The figure shows three views and two pictorial views of one solid part (mm, origin at its lowest corner). Answer the questions. A direction names the side the tool comes from. Round coordinates to 2 decimals unless told otherwise and drop trailing zeros. Write each loop counter-clockwise with the first axis right and the second up, starting at its lowest first coordinate (ties: lowest second). Pieces come first, ordered by that corner, then holes.
Item 1: Find section C-C on y = 20.25. Give the vertices of the cut face in (x, z) (1 decimal).
Item 2: For a pull along Y with two mould halves and no side action, classify the marked faces 1, 2, 3 and 4 as +Y half, -Y half, draft (parallel to the pull), parting line (faces both ways), or undercut.
Item 3: Find the intervals of material crossed by probe 1 along Y at (x, z) = (3.81, 1.25); probe 2 along X at (y, z) = (9.75, 10) (1 decimal); probe 3 along X at (y, z) = (10.5, 3.75) (1 decimal), in increasing order.
Item 4: Each of these flat-tipped pins is pushed along its axis until it touches: pin 1 (2.5 mm diameter, centred on x = 3.81, y = 5.4, fed in from -Z); pin 2 (1.5 mm diameter, centred on x = 31, y = 10, fed in from +Z); pin 3 (4 mm diameter, centred on y = 11.5, z = 13.5, fed in from -X). Where does it stop, or does it pass through?
Item 5: Find section B-B on x = 3.81. Give the vertices of the cut face in (y, z).
Item 6: Find section A-A on z = 8.25. Give the vertices of the cut face in (x, y) (1 decimal), then the cut area to 3 significant figures.
Item 7: Find section D-D on x = 30.5. Give the vertices of the cut face in (y, z), then the cut area to 3 significant figures.
Item 8: A tool of negligible diameter and unlimited length cuts with its end or side. For the marked faces 5, 6 and 7, from which of +Z, -Z, +X, -X, +Y, -Y can it reach the whole face along a straight path? Write none if from no direction.
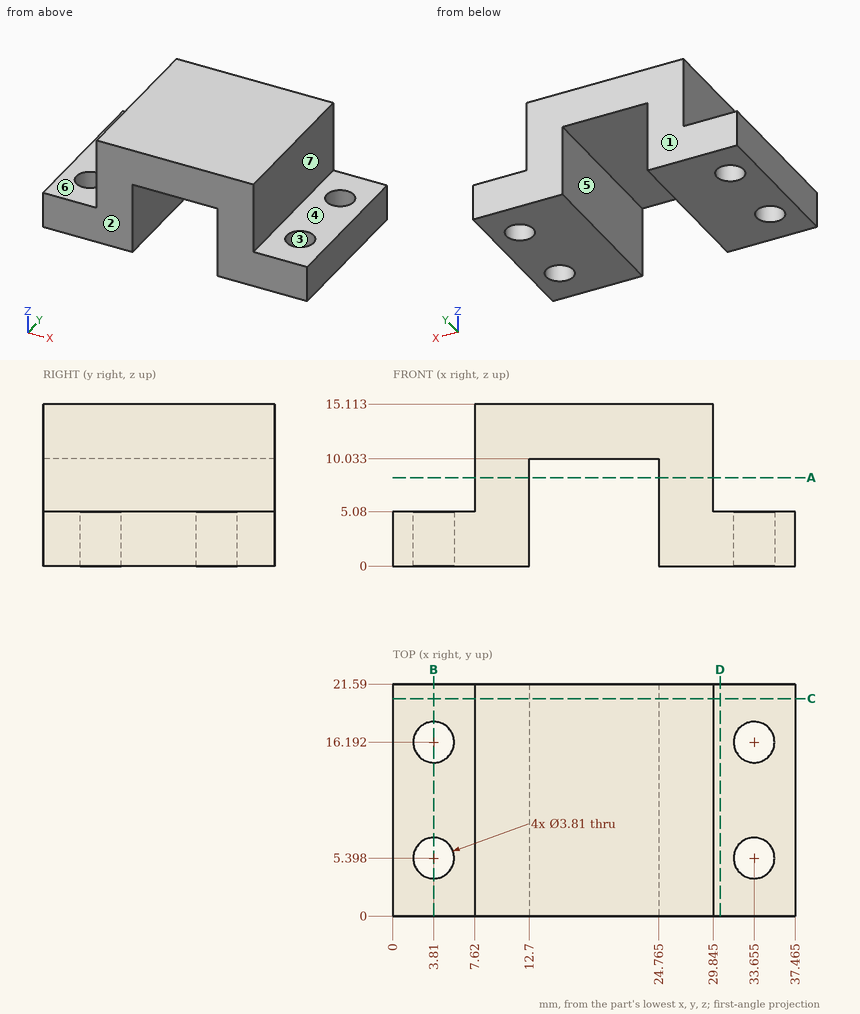
Check values:
1. outline: (0, 0) - (12.7, 0) - (12.7, 10) - (24.8, 10) - (24.8, 0) - (37.5, 0) - (37.5, 5.1) - (29.8, 5.1) - (29.8, 15.1) - (7.6, 15.1) - (7.6, 5.1) - (0, 5.1) - close
2. face 1: +Y half
2. face 2: -Y half
2. face 3: undercut
2. face 4: draft
3. probe 1: y = 0 to 3.49, 7.3 to 14.29, 18.1 to 21.59
3. probe 2: x = 7.6 to 12.7, 24.8 to 29.8
3. probe 3: x = 0 to 12.7, 24.8 to 37.5
4. pin 1: passes through
4. pin 2: stops at z = 5.08
4. pin 3: stops at x = 7.62
5. outline: (0, 0) - (3.49, 0) - (3.49, 5.08) - (0, 5.08) - close; (7.3, 0) - (14.29, 0) - (14.29, 5.08) - (7.3, 5.08) - close; (18.1, 0) - (21.59, 0) - (21.59, 5.08) - (18.1, 5.08) - close
6. outline: (7.6, 0) - (12.7, 0) - (12.7, 21.6) - (7.6, 21.6) - close; (24.8, 0) - (29.8, 0) - (29.8, 21.6) - (24.8, 21.6) - close
6. area: 219 mm2
7. outline: (0, 0) - (21.59, 0) - (21.59, 5.08) - (0, 5.08) - close
7. area: 110 mm2
8. face 5: -Z, +Y, -Y
8. face 6: +Z, -X, +Y, -Y
8. face 7: +Z, +X, +Y, -Y
